Design review of the part built by this model. Coordinates are the model's own, in mm. Round coordinates to 2 decimals unless told otherwise and drop trailing zeros. Order: outer loops, then holes, each group sorted by start corner. A loop starts at its lowest first (then second) coordinate and runs counter-clockwise, first axis right, second up. Notation, with made-up numbers: M 0,-7 L 19,-7 A7 cw 19,6 Z; hole C -19,33 d7. An arc over 180 degrees is marked long. Use a Markdown table: item, result. Add a question column.
(1) Take a section at C-C (y = -8.75). Write out the cut boundary in (x, z).
(2) Take a section at B-B (z = -4.5). Write out the cut boundary in (x, y).
(3) Take a section at A-A (x = 30.5). Write out the cut boundary in (y, z).
(4) Take a section at D-D (x = -30). Write out the cut boundary in (y, z).
(5) The part is to be moulded in two halves that separate along Z. For faces 1 (the face through (-8.829, -7.395, 17.497)), 2 (the face through (-51.095, -7.395, 0.184)), 3 (the face through (57.52, -7.4, 9.01)), say which applies: released by +Z, released by -Z, zero draft, split by the parting line, or undercut.
(6) For pin 1 (1.5 mm diameter, centred on y = -2, z = -14.5, fed in from -X); pin 2 (2 mm diameter, centred on x = 23, y = -13, fed in from +Z); pin 3 (2 mm diameter, centred on x = 6.5, y = -10, fed in from +Z), all flat-tipped, find the tip position at first contact; note any pin that passes through.
(7) To check wall thickness, follow probe 1 along X at (y, z) = (-10, -3.5); probe 2 along X at (y, z) = (-7.75, 5); probe 3 along Z at (x, y) = (22, -11.25). State the ranges of each line that lie inside material, in increasing order. Write a range as from..to.
```python
from build123d import *

# Parameters (mm, degrees)
F0_R     = 15
F0_R_2   = 30
F1_DEPTH = 15


with BuildPart() as f1:
    # F0 (on Front) → F1 (new body)
    with BuildSketch(Plane.XZ):
        with BuildLine():
            ThreePointArc((-23.175316, -18.364728), (-14.386495, -10.990608), (-11.09597, 0))
            ThreePointArc((-11.09597, 0), (-14.589644, 11.293415), (-23.850092, 18.641278))
            ThreePointArc((-23.850092, 18.641278), (-51.092646, -0.364624), (-23.175316, -18.364728))
        make_face()
        with Locations((-31.09597, 0)):
            Circle(F0_R, mode=Mode.SUBTRACT)
        with BuildLine():
            ThreePointArc((-23.850092, 18.641278), (-14.589644, 11.293415), (-11.09597, 0))
            ThreePointArc((-11.09597, 0), (-14.386495, -10.990608), (-23.175316, -18.364728))
            ThreePointArc((-23.175316, -18.364728), (-9.042619, -16.937632), (3.337154, -23.902611))
            ThreePointArc((3.337154, -23.902611), (-6.092708, 0.477784), (3.99921, 24.591664))
            ThreePointArc((3.99921, 24.591664), (-9.035618, 17.451877), (-23.850092, 18.641278))
        make_face()
        with BuildLine():
            ThreePointArc((63.90403, 0), (42.195593, 32.377992), (3.99921, 24.591664))
            ThreePointArc((3.99921, 24.591664), (-6.092708, 0.477784), (3.337154, -23.902611))
            ThreePointArc((3.337154, -23.902611), (41.752363, -32.556418), (63.90403, 0))
        make_face()
        with Locations((28.90403, 0)):
            Circle(F0_R_2, mode=Mode.SUBTRACT)
    extrude(amount=F1_DEPTH)


solid = f1.part
```
Verdict:
| question | item | result |
|---|---|---|
| 1 | outline | M -23.85,18.64 A20 ccw long -23.18,-18.36 A23.53 cw 3.34,-23.9 A35 ccw long 4,24.59 A25.93 cw Z; hole C -31.1,0 d30; hole C 28.9,0 d60 |
| 2 | outline | M -50.58,-15 L -45.41,-15 L -45.41,0 L -50.58,0 Z; M -16.79,-15 L -0.76,-15 L -0.76,0 L -16.79,0 Z; M 58.56,-15 L 63.61,-15 L 63.61,0 L 58.56,0 Z |
| 3 | outline | M -15,-34.96 L 0,-34.96 L 0,-29.96 L -15,-29.96 Z; M -15,29.96 L 0,29.96 L 0,34.96 L -15,34.96 Z |
| 4 | outline | M -15,-19.97 L 0,-19.97 L 0,-14.96 L -15,-14.96 Z; M -15,14.96 L 0,14.96 L 0,19.97 L -15,19.97 Z |
| 5 | face 1 | released by +Z |
| 5 | face 2 | split by the parting line |
| 5 | face 3 | undercut |
| 6 | pin 1 | stops at x = -45.62 |
| 6 | pin 2 | stops at z = 34.65 |
| 6 | pin 3 | stops at z = 27.69 |
| 7 | probe 1 | x = -50.79..-45.68, -16.51..-0.89, 58.7..63.73 |
| 7 | probe 2 | x = -50.46..-45.24, -16.95..-0.68, 58.48..63.55 |
| 7 | probe 3 | z = -34.31..-29.19, 29.19..34.31 |
